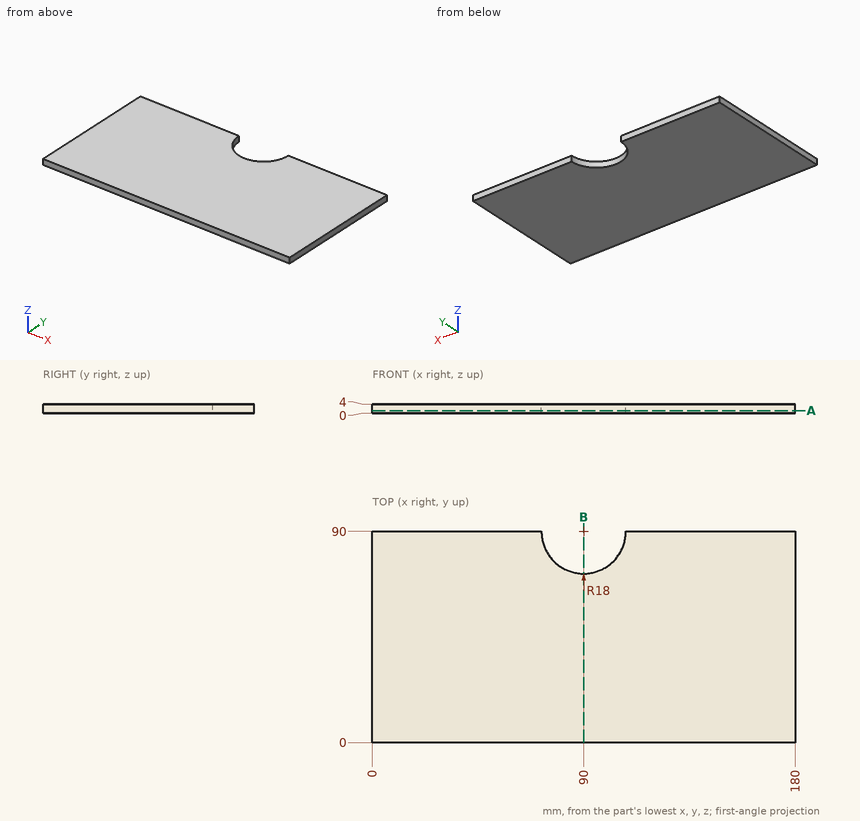
Source: three-view drawing plus pictorial views. Frame: mm from the lowest corner of the part. Round coordinates to 2 decimals unless told otherwise and drop trailing zeros. Loops run counter-clockwise (first coordinate to the right, second up) from the corner with the lowest first, then second, coordinate; pieces in that order, holes last.
Q1. Section B-B on x = 90. Return loops of the section in (y, z), plus the area to 3 significant figures.
Q2. Section A-A on z = 1.2. Return loops of the section in (x, y).
Q3. Material intervals for L1, parallel to Y at x = 79.5, z = 1.85; L2, parallel to Y at x = 86.5, z = 1.15, sorted ascending.
Evaluation:
1. outline: (0, 0) - (72, 0) - (72, 4) - (0, 4) - close
1. area: 288 mm2
2. outline: (0, 0) - (180, 0) - (180, 90) - (108, 90) arc R18 cw to (72, 90) - (0, 90) - close
3. L1: y = 0 to 75.38
3. L2: y = 0 to 72.34
